Geometry check sheet. Reference: drawing and pictorial views, mm from the part's lowest x, y, z. Coordinates: 2 decimals unless noted, no trailing zeros. Loops run counter-clockwise (first coordinate to the right, second up) from the corner with the lowest first, then second, coordinate; pieces in that order, holes last. Notation, with made-up numbers: (-20.75, -34) -> (24.25, -34) arc R20 cw to (24.25, 3) -> close; hole circle Ø2 at (63, 23). An arc over 180 degrees is marked (long way). Answer as a JSON object with one key per item and string values. Group by question number.
Q1. Cross-section at D-D on z = 6. Record the boundary of the cut face in (x, y).
Q2. Scan lines: L1, parallel to Z at x = 4, y = 4 (1 decimal); L2, parallel to Z at x = 5, y = 2.5 (1 decimal); L3, parallel to Y at x = 3.75, z = 26 (1 decimal). Record each from-to range of solid material in increasing order.
Q3. Cross-section at C-C on x = 7. Record the boundary of the cut face in (y, z), and give its area (3 significant figures).
Q4. Gauge pin test, flat ends, axial feed: pin 1 Ø2 at (y, z) = (2.5, 74) entering from +X; pin 2 Ø3.5 at (x, z) = (3.95, 3.18) entering from +Y; pin 3 Ø1.6 at (x, z) = (3.95, 88.27) entering from -Y. Record the tip position at first contact, or that the pin passes through.
Q5. Cross-section at A-A on y = 5. Give the number of separate pieces and of enclosed holes in the cut face.
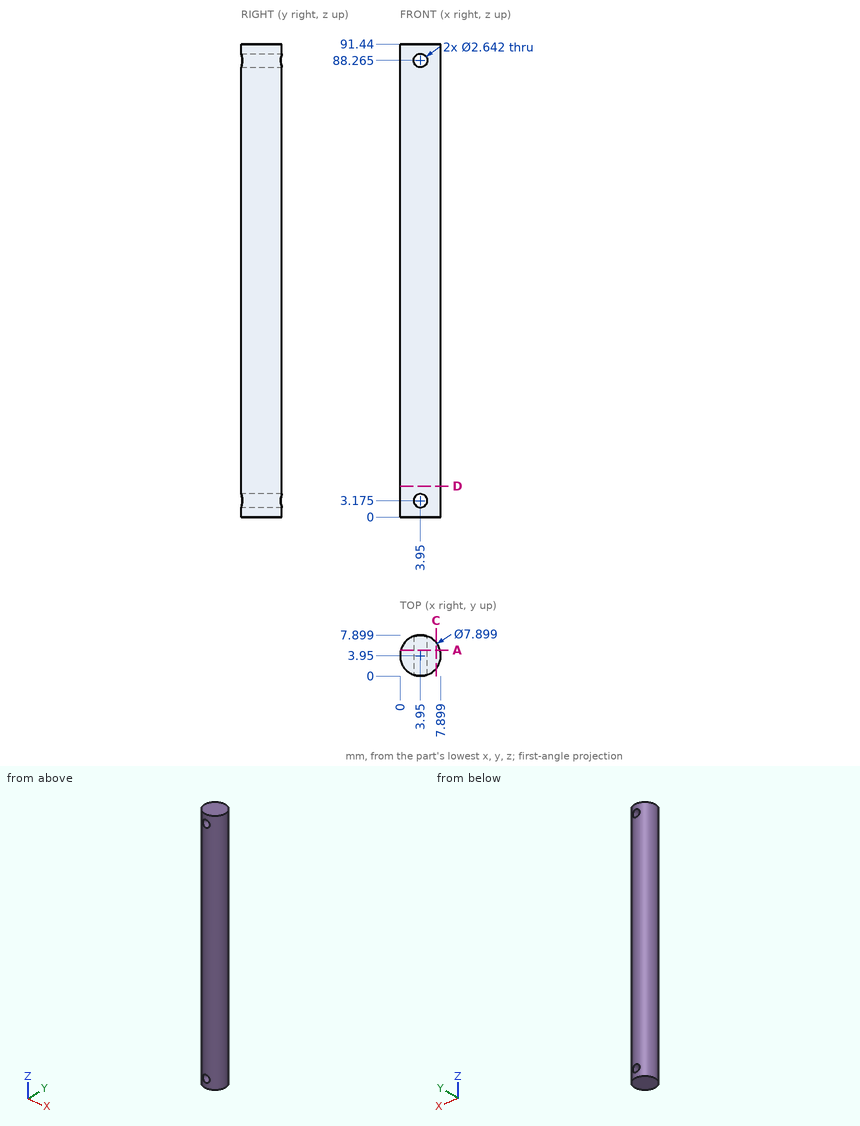
Computed values:
{
 "1": {"outline": "circle Ø7.9 at (3.95, 3.95)"},
 "2": {"L1": "z = 0 to 1.9, 4.5 to 86.9, 89.6 to 91.4", "L2": "z = 0 to 2.4, 4 to 87.5, 89.1 to 91.4", "L3": "y = 0 to 7.9"},
 "3": {"outline": "(1.44, 0) -> (6.46, 0) -> (6.46, 91.44) -> (1.44, 91.44) -> close", "area": "459 mm²"},
 "4": {"pin 1": "stops at x = 7.87", "pin 2": "stops at y = 7.9", "pin 3": "passes through"},
 "5": {"separate pieces": "1", "enclosed holes": "2"}
}
